Drawing for the job (mm, zero at the part's lowest x, y, z). A direction names the side the tool comes from. Give positions to 0.01 mm unless a question says otherwise; leave off trailing zeros. Order: outer loops, then holes, each group sorted by start corner. A loop starts at its lowest first (then second) coordinate and runs counter-clockwise, first axis right, second up. Notation, with made-up numbers: (6, 71.5) - (12, 71.5) arc R32 cw to (12, 102.5) - close; hole circle Ø4 at (-14.5, 18.25). An arc over 180 degrees is marked (long way). One line per item, written item: value.
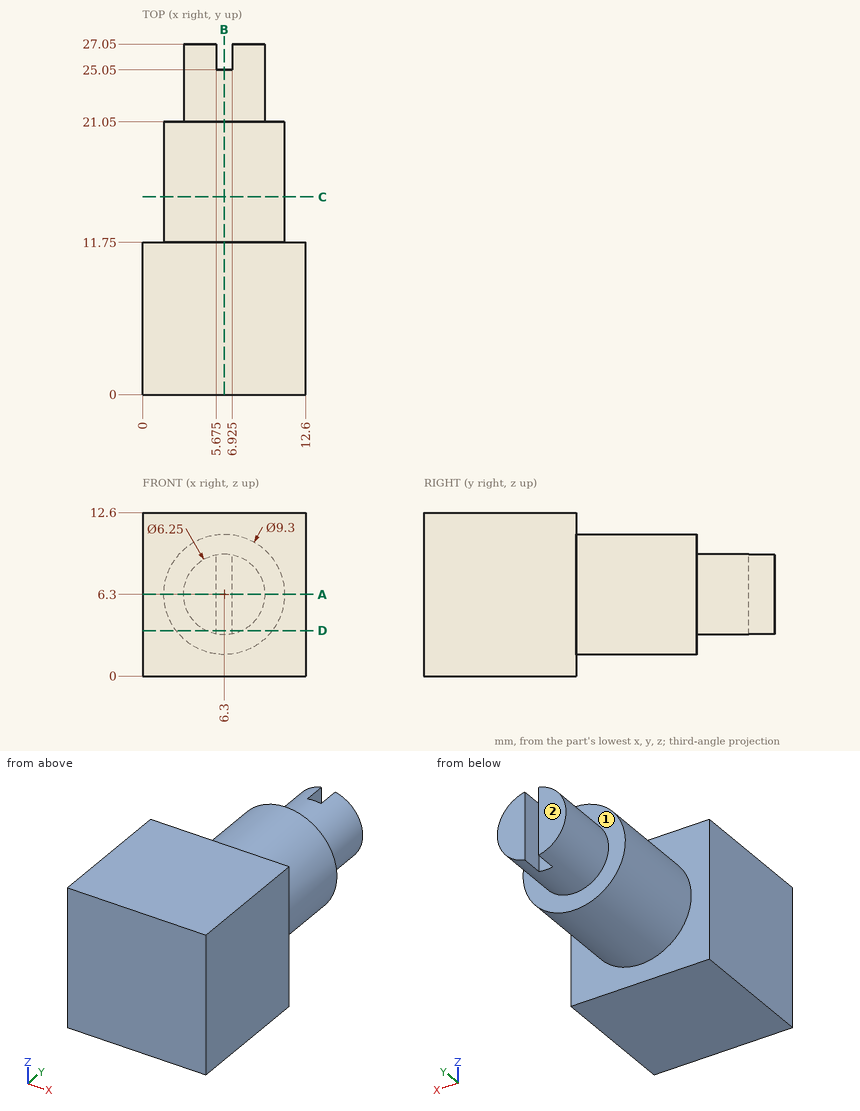
(1) Pin check, flat tips, straight feed: P1, Ø1, axis at x = 9, y = 17.5, coming from the +Z side; P2, Ø3, axis at y = 23, z = 9, coming from the +X side; P3, Ø1.6, axis at y = 26, z = 6.5, coming from the +X side (3 decimals). Stop position of each tip, or through.
Completed:
P1: z = 10.4
P2: x = 9.19
P3: x = 9.425
(2) Slice it at D-D, the plane z = 3.5. Give the cut face in (x, y) (3 decimals).
Completed:
outline: (0, 0) - (12.6, 0) - (12.6, 11.75) - (10.012, 11.75) - (10.012, 21.05) - (7.688, 21.05) - (7.688, 27.05) - (6.925, 27.05) - (6.925, 25.05) - (5.675, 25.05) - (5.675, 27.05) - (4.912, 27.05) - (4.912, 21.05) - (2.588, 21.05) - (2.588, 11.75) - (0, 11.75) - close
(3) Slice it at A-A, the plane z = 6.3. Give the cut face in (x, y) (3 decimals).
Completed:
outline: (0, 0) - (12.6, 0) - (12.6, 11.75) - (10.95, 11.75) - (10.95, 21.05) - (9.425, 21.05) - (9.425, 27.05) - (6.925, 27.05) - (6.925, 25.05) - (5.675, 25.05) - (5.675, 27.05) - (3.175, 27.05) - (3.175, 21.05) - (1.65, 21.05) - (1.65, 11.75) - (0, 11.75) - close
(4) Drill centre lines: line 1 (Y direction, x = 11.25, z = 1); line 2 (Z direction, x = 4.5, y = 12.5); line 3 (Y direction, x = 9.25, z = 3.5). Where is each one in solid material? Low to high.
Completed:
line 1: 0 to 11.75
line 2: 2.01 to 10.59
line 3: 0 to 21.05
(5) Slice it at C-C, the plane y = 15.25. Give the cut face in (x, z), and give its area (3 significant figures).
Completed:
outline: circle Ø9.3 at (6.3, 6.3)
area: 67.9 mm²
(6) Slice it at B-B, the plane x = 6.3. Give the cut face in (y, z) (3 decimals).
Completed:
outline: (0, 0) - (11.75, 0) - (11.75, 1.65) - (21.05, 1.65) - (21.05, 3.175) - (25.05, 3.175) - (25.05, 9.425) - (21.05, 9.425) - (21.05, 10.95) - (11.75, 10.95) - (11.75, 12.6) - (0, 12.6) - close
(7) 3-axis set-ups, long thin cutter, end or side, ignore diameter. For the marked faces 1 and 2: which of +Z, -Z, +X, -X, +Y, -Y reach the whole face in a straight line?
Completed:
face 1: +Y
face 2: +Z, -Z, +X, -X, +Y
